The listing builds one solid part. Answer for the finished solid, in the listing's coordinates (mm). Coordinates: 2 decimals unless noted, no trailing zeros. Loops run counter-clockwise (first coordinate to the right, second up) from the corner with the lowest first, then second, coordinate; pieces in that order, holes last. Notation, with made-up numbers: M 75.5,44 L 87.5,44 A25 ccw 87.5,60 Z; hole C 9.25,25.5 d6. An arc over 180 degrees is marked long. Return JSON: item names as keys, results as strings. Group by question number.
1. Section A-A (x = 0) is taken. Write down the section's boundary in (y, z), then the cut area to 4 significant figures.
2. The mould has two halves that part along X. Classify faces 1 (the face through (7.5, -37, 3)), 2 (the face through (0, 3.5, 3)), 3 (the face through (0, 2, 3)): pulls with the +X half, pulls with the -X half, needs draft (parallel to the pull), parting line crosses it, or undercut.
3. Section B-B (y = 0) is taken. Write down the section's boundary in (x, z), then the cut area to 3 significant figures.
4. Straight lines are drawn through the part: L1, parallel to Y at x = 0, z = 3.25; L2, parallel to Y at x = 1.75, z = 0.5; L3, parallel to Y at x = 7, z = 4.75. For each, find the intervals that lie inside material, in ascending order. Write a range as from..to.
Autodesk Inventor part; units mm, degrees
ref_plane "YZ Plane" through (0, 0, 0) normal (1, 0, 0) x (0, 1, 0)
ref_plane "XZ Plane" through (0, 0, 0) normal (0, 1, 0) x (-1, 0, 0)
ref_plane "XY Plane" through (0, 0, 0) normal (0, 0, 1) x (1, 0, 0)
sketch "Sketch1" plane through (0, 0, 0) normal (0, 0, 1) x (1, 0, 0)
  circle A0 centre (0, 0) radius 2
  line L0 (-5.5, 3.5) -> (5.5, 3.5)
  line L1 (7.5, 1.5) -> (7.5, -3.5)
  line L2 (7.5, -3.5) -> (-7.5, -3.5)
  line L3 (-7.5, -3.5) -> (-7.5, 1.5)
  arc A1 (-5.5, 3.5) -> (-7.5, 1.5) centre (-5.5, 1.5) ccw
  arc A2 (7.5, 1.5) -> (5.5, 3.5) centre (5.5, 1.5) ccw
  point P0 (7.5, 3.5)
  dimension "d0" = 4
  dimension "d1" = 15
  dimension "d2" = 7
  dimension "d3" = 7.5
  dimension "d4" = 3.5
  dimension "d5" = 2
extrude "Extrusion1" add sketch "Sketch1" along normal blind 7
sketch "Sketch2" plane through (-7.5, -3.5, 0) normal (0, -1, 0) x (1, 0, 0)
  line L0 (15, 0) -> (13, 0)
  line L1 (0, 7) -> (15, 7)
  line L2 (15, 7) -> (15, 0)
  line L3 (15, 0) -> (0, 0)
  line L4 (0, 0) -> (0, 7)
  line L5 (0, 7) -> (15, 7)
  line L6 (0, 0) -> (0, 7)
  point P0 (7.5, 0)
  dimension "d8" = 0
  dimension "d9" = 0
extrude "Extrusion2" add sketch "Sketch2" along normal blind 73.5
properties part number "backside arm"
Worked out:
{
 "1": {"outline": "M -77,0 L -2,0 L -2,7 L -77,7 Z; M 2,0 L 3.5,0 L 3.5,7 L 2,7 Z", "area": "535.5 mm^2"},
 "2": {"face 1": "pulls with the +X half", "face 2": "needs draft", "face 3": "undercut"},
 "3": {"outline": "M -7.5,0 L -2,0 L -2,7 L -7.5,7 Z; M 2,0 L 7.5,0 L 7.5,7 L 2,7 Z", "area": "77.0 mm^2"},
 "4": {"L1": "-77..-2, 2..3.5", "L2": "-77..-0.97, 0.97..3.5", "L3": "-77..2.82"}
}
